from build123d import *

# Parameters (mm, degrees)
SKETCH_2_R      = 1.6
SKETCH_2_R_2    = 2.1
EXTRUDE_3_DEPTH = 5
FILLET_1_R      = 4
FILLET_2_R      = 10
FILLET_3_R      = 2


with BuildPart() as part:
    # 草图2 → 凸台-拉伸3 (new body)
    with BuildSketch(Plane.XY):
        Polygon((-53, 20), (53, 20), (53, 35.656854249), (61.920310217, 44.577164466), (67.577164466, 38.920310217), (60, 31.34314575), (60, 20), (60, -20), (-60, -20), (-60, 20), (-60, 31.34314575), (-67.577164466, 38.920310217), (-61.920310217, 44.577164466), (-53, 35.656854249), align=None)
        with Locations((-56, 17)):
            Circle(SKETCH_2_R, mode=Mode.SUBTRACT)
        with Locations((-48, 17)):
            Circle(SKETCH_2_R, mode=Mode.SUBTRACT)
        with Locations((-40, 17)):
            Circle(SKETCH_2_R, mode=Mode.SUBTRACT)
        with Locations((-32, 17)):
            Circle(SKETCH_2_R, mode=Mode.SUBTRACT)
        with Locations((-24, 17)):
            Circle(SKETCH_2_R, mode=Mode.SUBTRACT)
        with Locations((-16, 17)):
            Circle(SKETCH_2_R, mode=Mode.SUBTRACT)
        with Locations((-8, 17)):
            Circle(SKETCH_2_R, mode=Mode.SUBTRACT)
        with Locations((0, 17)):
            Circle(SKETCH_2_R, mode=Mode.SUBTRACT)
        with Locations((8, 17)):
            Circle(SKETCH_2_R, mode=Mode.SUBTRACT)
        with Locations((16, 17)):
            Circle(SKETCH_2_R, mode=Mode.SUBTRACT)
        with Locations((24, 17)):
            Circle(SKETCH_2_R, mode=Mode.SUBTRACT)
        with Locations((32, 17)):
            Circle(SKETCH_2_R, mode=Mode.SUBTRACT)
        with Locations((40, 17)):
            Circle(SKETCH_2_R, mode=Mode.SUBTRACT)
        with Locations((48, 17)):
            Circle(SKETCH_2_R, mode=Mode.SUBTRACT)
        with Locations((56, 17)):
            Circle(SKETCH_2_R, mode=Mode.SUBTRACT)
        with Locations((-62.627416998, 39.627416998)):
            Circle(SKETCH_2_R, mode=Mode.SUBTRACT)
        with Locations(Location((62.627416998, 39.627416998, 0), (0, 0, 180))):
            Circle(SKETCH_2_R, mode=Mode.SUBTRACT)
        with Locations((-56, 9)):
            Circle(SKETCH_2_R, mode=Mode.SUBTRACT)
        with Locations((-48, 9)):
            Circle(SKETCH_2_R, mode=Mode.SUBTRACT)
        with Locations((-40, 9)):
            Circle(SKETCH_2_R, mode=Mode.SUBTRACT)
        with Locations((-32, 9)):
            Circle(SKETCH_2_R, mode=Mode.SUBTRACT)
        with Locations((-24, 9)):
            Circle(SKETCH_2_R, mode=Mode.SUBTRACT)
        with Locations((-16, 9)):
            Circle(SKETCH_2_R, mode=Mode.SUBTRACT)
        with Locations((-8, 9)):
            Circle(SKETCH_2_R, mode=Mode.SUBTRACT)
        with Locations((0, 9)):
            Circle(SKETCH_2_R, mode=Mode.SUBTRACT)
        with Locations((8, 9)):
            Circle(SKETCH_2_R, mode=Mode.SUBTRACT)
        with Locations((16, 9)):
            Circle(SKETCH_2_R, mode=Mode.SUBTRACT)
        with Locations((24, 9)):
            Circle(SKETCH_2_R, mode=Mode.SUBTRACT)
        with Locations((32, 9)):
            Circle(SKETCH_2_R, mode=Mode.SUBTRACT)
        with Locations((40, 9)):
            Circle(SKETCH_2_R, mode=Mode.SUBTRACT)
        with Locations((48, 9)):
            Circle(SKETCH_2_R, mode=Mode.SUBTRACT)
        with Locations((56, 9)):
            Circle(SKETCH_2_R, mode=Mode.SUBTRACT)
        with Locations((-56, -16)):
            Circle(SKETCH_2_R_2, mode=Mode.SUBTRACT)
        with Locations((-56, -8)):
            Circle(SKETCH_2_R_2, mode=Mode.SUBTRACT)
        with Locations((-56, 0)):
            Circle(SKETCH_2_R_2, mode=Mode.SUBTRACT)
        with Locations(Location((56, -16, 0), (0, 0, 180))):
            Circle(SKETCH_2_R_2, mode=Mode.SUBTRACT)
        with Locations(Location((56, -8, 0), (0, 0, 180))):
            Circle(SKETCH_2_R_2, mode=Mode.SUBTRACT)
        with Locations(Location((56, 0, 0), (0, 0, 180))):
            Circle(SKETCH_2_R_2, mode=Mode.SUBTRACT)
        with Locations((-56.970562748, 33.970562748)):
            Circle(SKETCH_2_R, mode=Mode.SUBTRACT)
        with Locations(Location((56.970562748, 33.970562748, 0), (0, 0, 180))):
            Circle(SKETCH_2_R, mode=Mode.SUBTRACT)
        with BuildLine():
            Line((-20, -7.9), (20, -7.9))
            ThreePointArc((20, -7.9), (22.1, -10), (20, -12.1))
            Line((20, -12.1), (-20, -12.1))
            ThreePointArc((-20, -12.1), (-22.1, -10), (-20, -7.9))
        make_face(mode=Mode.SUBTRACT)
    extrude(amount=EXTRUDE_3_DEPTH)

    # 圆角1
    fillet_1_edges = [part.edges().sort_by_distance(p)[0] for p in [
        (60, -20, 2.5),
        (-60, -20, 2.5),
        (-53, 35.656854249, 2.5),
        (53, 35.656854249, 2.5),
    ]]
    fillet(fillet_1_edges, radius=FILLET_1_R)

    # 圆角2
    fillet_2_edges = [part.edges().sort_by_distance(p)[0] for p in [
        (-60, 31.34314575, 2.5),
        (60, 31.34314575, 2.5),
    ]]
    fillet(fillet_2_edges, radius=FILLET_2_R)

    # 圆角3
    fillet_3_edges = [part.edges().sort_by_distance(p)[0] for p in [
        (-67.577164466, 38.920310217, 2.5),
        (-61.920310217, 44.577164466, 2.5),
        (61.920310217, 44.577164466, 2.5),
        (67.577164466, 38.920310217, 2.5),
    ]]
    fillet(fillet_3_edges, radius=FILLET_3_R)


solid = part.part
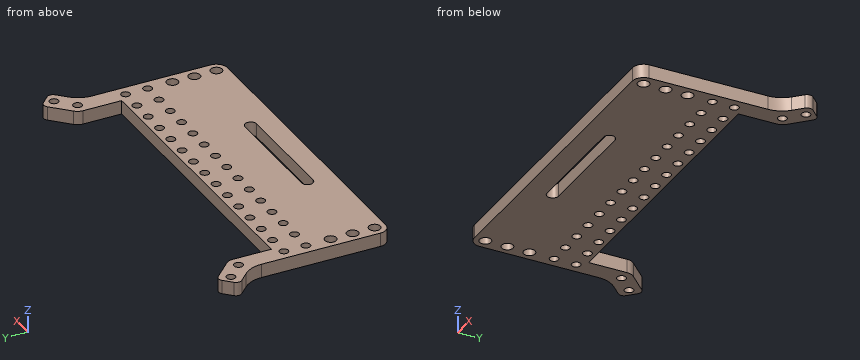
CAD build for the part. Positions are in the model's coordinates, mm. Round coordinates to 2 decimals unless told otherwise and drop trailing zeros. Loops run counter-clockwise (first coordinate to the right, second up) from the corner with the lowest first, then second, coordinate; pieces in that order, holes last. Notation, with made-up numbers: M 14,-11 L 57,-11 A18 cw 57,17 Z; hole C -8,32 d5. An arc over 180 degrees is marked long. One line per question, with ' | ' between items. Start each with the question number.
Item 1: Pin check, flat tips, straight feed: pin 1 Ø1.9 at (x, y) = (56, 17) entering from -Z; pin 2 Ø3.5 at (x, y) = (-16, 17) entering from -Z; pin 3 Ø1 at (x, z) = (-50.5, 3) entering from +Y; pin 4 Ø2.5 at (y, z) = (14, 1.5) entering from -X. Stop position of each tip, or through.
Item 2: Cut at C-C, the plane x = -13. Write the cut outline in (y, z), plus the area to 3 significant figures.
Item 3: Wall check: line 1 (Y direction, x = 8, z = 3.55); line 2 (Y direction, x = -48, z = 1.05); line 3 (X direction, y = 34, z = 4.2). Give the ranges that are in metal, low to high.
Item 4: Cut at A-A, the plane x = 8. Write the cut outline in (y, z).
Item 5: Cut at D-D, the plane x = 48. Write the cut outline in (y, z).
Item 6: Cut at B-B, the plane y = 23. Write the cut outline in (x, z).
Responses:
1) pin 1: passes through | pin 2: stops at z = 0 | pin 3: stops at y = 20 | pin 4: stops at x = -60
2) outline: M -20,0 L -12.1,0 L -12.1,5 L -20,5 Z; M -7.9,0 L 20,0 L 20,5 L -7.9,5 Z | area: 179 mm²
3) line 1: y = -20 to -12.1, -7.9 to 7.4, 10.6 to 15.4, 18.6 to 20 | line 2: y = -20 to 7.4, 10.6 to 15.4, 18.6 to 20 | line 3: x = -62.67 to -58.57, -55.37 to -53, 53 to 55.37, 58.57 to 62.67
4) outline: M -20,0 L -12.1,0 L -12.1,5 L -20,5 Z; M -7.9,0 L 7.4,0 L 7.4,5 L -7.9,5 Z; M 10.6,0 L 15.4,0 L 15.4,5 L 10.6,5 Z; M 18.6,0 L 20,0 L 20,5 L 18.6,5 Z
5) outline: M -20,0 L 7.4,0 L 7.4,5 L -20,5 Z; M 10.6,0 L 15.4,0 L 15.4,5 L 10.6,5 Z; M 18.6,0 L 20,0 L 20,5 L 18.6,5 Z
6) outline: M -60,0 L -53,0 L -53,5 L -60,5 Z; M 53,0 L 60,0 L 60,5 L 53,5 Z
